Check sheet for the modelled part. Datum: model origin and axes. Units: mm. A direction names the side the tool comes from. Round coordinates to 2 decimals unless told otherwise and drop trailing zeros. Order: outer loops, then holes, each group sorted by start corner. A loop starts at its lowest first (then second) coordinate and runs counter-clockwise, first axis right, second up.
Autodesk Inventor part; units mm, degrees
ref_plane "YZ Plane" through (0, 0, 0) normal (1, 0, 0) x (0, 1, 0)
ref_plane "XZ Plane" through (0, 0, 0) normal (0, 1, 0) x (-1, 0, 0)
ref_plane "XY Plane" through (0, 0, 0) normal (0, 0, 1) x (1, 0, 0)
sketch "Sketch1" plane through (0, 0, 0) normal (0, 1, 0) x (-1, 0, 0)
  line L0 (19.05, 38.1) -> (-19.05, 38.1)
  line L1 (-19.05, 38.1) -> (-19.05, -38.1)
  line L2 (-19.05, -38.1) -> (19.05, -38.1)
  line L3 (19.05, -38.1) -> (19.05, 38.1)
  point P0 (0, 0)
  point P1 (19.05, 0)
  point P2 (0, -38.1)
  dimension "d0" = 76.2
  dimension "d1" = 38.1
extrude "Extrusion1" add sketch "Sketch1" along normal blind 4
sketch "Sketch2" plane through (19.05, 0, 38.1) normal (1, 0, 0) x (0, 0, -1)
  line L0 (5.08, 3.143) -> (12.446, 3.143)
  line L1 (12.446, 3.143) -> (12.446, 0.857)
  line L2 (12.446, 0.857) -> (5.08, 0.857)
  line L3 (5.08, 0.857) -> (5.08, 3.143)
  line L4 (0, 0) -> (0, 4)
  line L5 (0, 4) -> (76.2, 4)
  line L6 (17.526, 3.143) -> (24.892, 3.143)
  line L7 (24.892, 3.143) -> (24.892, 0.857)
  line L8 (24.892, 0.857) -> (17.526, 0.857)
  line L9 (17.526, 0.857) -> (17.526, 3.143)
  line L10 (29.972, 3.143) -> (37.338, 3.143)
  line L11 (37.338, 3.143) -> (37.338, 0.857)
  line L12 (37.338, 0.857) -> (29.972, 0.857)
  line L13 (29.972, 0.857) -> (29.972, 3.143)
  line L14 (42.418, 3.143) -> (49.784, 3.143)
  line L15 (49.784, 3.143) -> (49.784, 0.857)
  line L16 (49.784, 0.857) -> (42.418, 0.857)
  line L17 (42.418, 0.857) -> (42.418, 3.143)
  line L18 (54.864, 3.143) -> (62.23, 3.143)
  line L19 (62.23, 3.143) -> (62.23, 0.857)
  line L20 (62.23, 0.857) -> (54.864, 0.857)
  line L21 (54.864, 0.857) -> (54.864, 3.143)
  point P0 (38.1, 0)
  point P1 (5.08, 2)
  point P2 (0, 2)
  point P3 (17.526, 2)
  point P4 (0, 2)
  point P5 (29.972, 2)
  point P6 (0, 2)
  point P7 (42.418, 2)
  point P8 (0, 2)
  dimension "d4" = 5.08
  dimension "d5" = 7.366
  dimension "d6" = 2.286
  dimension "d8" = 5.08
  dimension "d9" = 7.366
  dimension "d10" = 2.286
  dimension "d11" = 7.366
  dimension "d12" = 2.286
  dimension "d13" = 5.08
  dimension "d14" = 7.366
  dimension "d15" = 2.286
  dimension "d16" = 5.08
  dimension "d18" = 7.366
  dimension "d19" = 5.08
extrude "Extrusion2" add sketch "Sketch2" along normal blind 5.08
sketch "Sketch4" plane through (0, 4, 0) normal (0, 1, 0) x (1, 0, 0)
  circle A0 centre (8.05, 27.1) radius 1.27
  line L0 (19.05, -38.1) -> (19.05, 38.1)
  line L1 (19.05, 38.1) -> (-19.05, 38.1)
  circle A1 centre (-11.95, 27.1) radius 1.27
  line L2 (-19.05, 38.1) -> (-19.05, -38.1)
  circle A2 centre (8.05, -29.796) radius 1.27
  circle A3 centre (-11.95, -29.796) radius 1.27
  line L3 (-19.05, -38.1) -> (19.05, -38.1)
  point P0 (0, 0)
  dimension "d27" = 11
  dimension "d28" = 11
  dimension "d31" = 2.54
  dimension "d32" = 2.54
  dimension "d37" = 2.54
  dimension "d38" = 2.54
  dimension "d41" = 20
  dimension "d42" = 56.896
  dimension "d43" = 56.896
extrude "Extrusion4" cut sketch "Sketch4" against normal blind 7.1628 contours A0 | A1 | A2 | A3
properties part number "pca"
Item 1: Access from +Z, -Z, +X, -X, +Y, -Y to the whole of each face (thin tool, end or side, straight path). Record for faces 1 (the flat face through (22, 0.857, -8)), 2 (the flat face through (22, 3.143, 4)), 3 (the cylindrical face through (7.114, 2.028, -27.958)), 4 (the flat face through (22, 2, -4.318)).
Answer:
face 1: +Z, -Z, +X, -Y
face 2: +Z, -Z, +X, +Y
face 3: +Y, -Y
face 4: +X, +Y, -Y
Item 2: Sectioned sample at D-D (z = 19). Record the cut outline in (x, y).
Answer:
outline: (-19.05, 0) - (19.05, 0) - (19.05, 0.86) - (24.13, 0.86) - (24.13, 3.14) - (19.05, 3.14) - (19.05, 4) - (-19.05, 4) - close
Item 3: Sectioned sample at A-A (x = 8.05). Record the cut outline in (y, z).
Answer:
outline: (0, -38.1) - (4, -38.1) - (4, -28.37) - (0, -28.37) - close; (0, -25.83) - (4, -25.83) - (4, 28.53) - (0, 28.53) - close; (0, 31.07) - (4, 31.07) - (4, 38.1) - (0, 38.1) - close
Item 4: Go/stop test with flat-tipped pins: P1, Ø0.7, axis at x = 21, y = 1.5, coming from the -Z side; P2, Ø3, axis at x = 4.5, z = -3.5, coming from the -Y side; P3, Ø1.1, axis at x = 23, y = 2.5, coming from the +Z side; P4, Ø2.5, axis at x = 21.5, z = 5, coming from the -Y side. Record where each tip stops, or that it passes through.
Answer:
P1: stops at z = -24.13
P2: stops at y = 0
P3: stops at z = 33.02
P4: stops at y = 0.86
Item 5: Sectioned sample at C-C (y = 1.9). Record the cut outline in (x, z), and give its area (3 significant figures).
Answer:
outline: (-19.05, -38.1) - (19.05, -38.1) - (19.05, -24.13) - (24.13, -24.13) - (24.13, -16.76) - (19.05, -16.76) - (19.05, -11.68) - (24.13, -11.68) - (24.13, -4.32) - (19.05, -4.32) - (19.05, 0.76) - (24.13, 0.76) - (24.13, 8.13) - (19.05, 8.13) - (19.05, 13.21) - (24.13, 13.21) - (24.13, 20.57) - (19.05, 20.57) - (19.05, 25.65) - (24.13, 25.65) - (24.13, 33.02) - (19.05, 33.02) - (19.05, 38.1) - (-19.05, 38.1) - close; hole circle Ø2.54 at (-11.95, -27.1); hole circle Ø2.54 at (-11.95, 29.8); hole circle Ø2.54 at (8.05, -27.1); hole circle Ø2.54 at (8.05, 29.8)
area: 3,070 mm2
Item 6: Sectioned sample at B-B (z = -27.1). Record the cut outline in (x, y), and give its area (3 significant figures).
Answer:
outline: (-19.05, 0) - (-13.22, 0) - (-13.22, 4) - (-19.05, 4) - close; (-10.68, 0) - (6.78, 0) - (6.78, 4) - (-10.68, 4) - close; (9.32, 0) - (19.05, 0) - (19.05, 4) - (9.32, 4) - close
area: 132 mm2
Item 7: Release check for a two-part mould opening along Z. For faces 5 (the flat face through (0, 4, 1)), 6 (the flat face through (22, 2, 13.208)), 7 (the flat face through (22, 2, 8.128)), 8 (the flat face through (0, 2, 38.1)) record: released by +Z, released by -Z, zero draft, split by the parting line, or undercut.
Answer:
face 5: zero draft
face 6: undercut
face 7: undercut
face 8: released by +Z
Item 8: Scan lines: line 1 along X through (y, z) = (1.25, -27.1); line 2 along Z through (x, y) = (19.5, 2.4); line 3 along Z through (x, y) = (-11.95, 1.55). Record each from-to range of solid material in increasing order.
Answer:
line 1: x = -19.05 to -13.22, -10.68 to 6.78, 9.32 to 19.05
line 2: z = -24.13 to -16.76, -11.68 to -4.32, 0.76 to 8.13, 13.21 to 20.57, 25.65 to 33.02
line 3: z = -38.1 to -28.37, -25.83 to 28.53, 31.07 to 38.1
